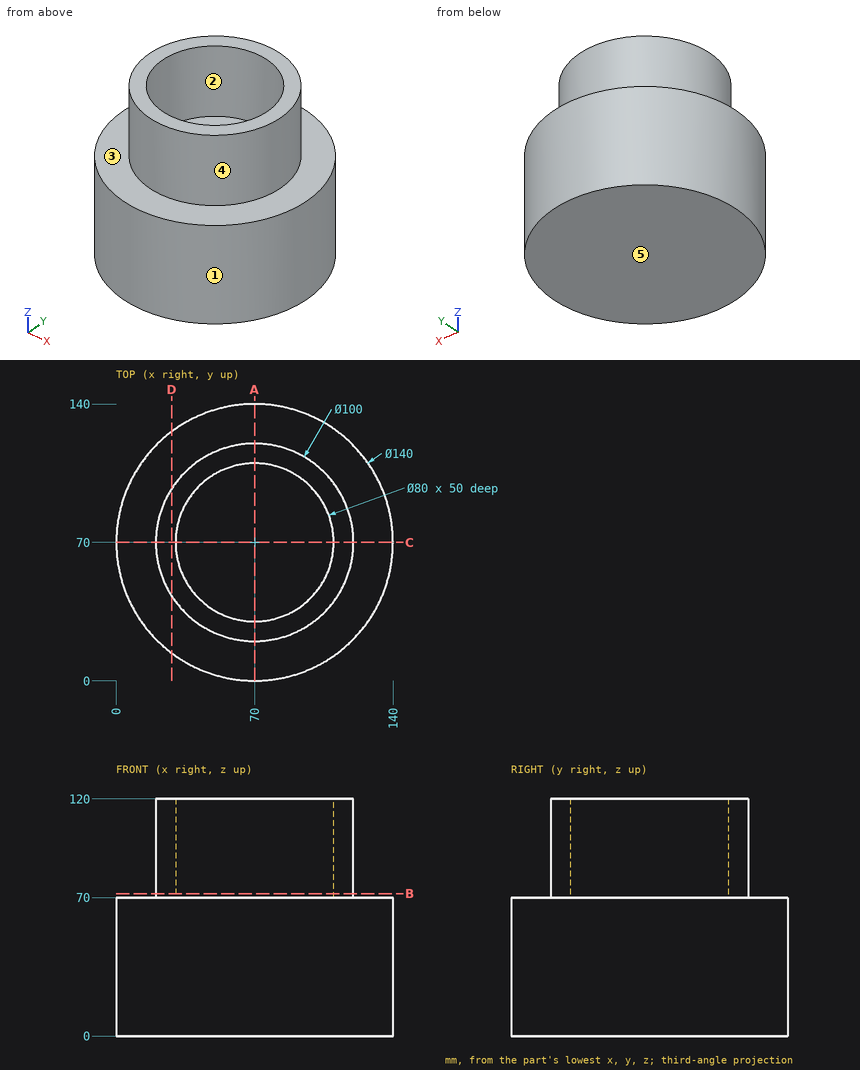
Can you work these out from the drawing? Everything is in mm from the part's minimum corner. A direction names the side the tool comes from. Round coordinates to 2 decimals unless told otherwise and drop trailing zeros. Write each loop counter-clockwise with the first axis right and the second up, starting at its lowest first coordinate (ties: lowest second). Pieces come first, ordered by that corner, then holes.
1. Will these pins go through, and if not, where does the flat tip stop? pin 1 Ø4 at (x, z) = (111.5, 60.5) entering from -Y; pin 2 Ø10 at (x, y) = (48, 78) entering from +Z; pin 3 Ø8 at (x, z) = (26.5, 92.5) entering from +Y.
2. Suppose I cut it at B-B (z = 72). List the corners of the cut face in (x, y) for me, and give its area (3 significant figures).
3. I need wall thicknesses on L1, parallel to Y at x = 70, z = 93; L2, parallel to Z at x = 71, y = 132; L3, parallel to X at y = 49, z = 87.5. Which ranges of each line are inside material? Lowest first, please.
4. If we mould it in two halves opening along Y, with no side actions, what happens to the marked faces 1, 2 and 3? For each: released by +Y, released by -Y, zero draft, split by the parting line, or undercut.
5. Suppose I cut it at D-D (x = 28). List the corners of the cut face in (y, z) for me, and give its area (3 significant figures).
6. For the marked faces 4 and 5, which set-ups out of +Z, -Z, +X, -X, +Y, -Y let a thin tool reach every point of the face, with its end or its side?
7. Suppose I cut it at A-A (x = 70). List the corners of the cut face in (y, z) for me.
Answer sheet:
1. pin 1: stops at y = 12.21
1. pin 2: stops at z = 70
1. pin 3: stops at y = 100.66
2. outline: circle Ø100 at (70, 70); hole circle Ø80 at (70, 70)
2. area: 2,830 mm2
3. L1: y = 20 to 30, 110 to 120
3. L2: z = 0 to 70
3. L3: x = 24.62 to 35.96, 104.04 to 115.38
4. face 1: split by the parting line
4. face 2: undercut
4. face 3: zero draft
5. outline: (14, 0) - (126, 0) - (126, 70) - (97.13, 70) - (97.13, 120) - (42.87, 120) - (42.87, 70) - (14, 70) - close
5. area: 10,600 mm2
6. face 4: +Z
6. face 5: -Z, +X, -X, +Y, -Y
7. outline: (0, 0) - (140, 0) - (140, 70) - (120, 70) - (120, 120) - (110, 120) - (110, 70) - (30, 70) - (30, 120) - (20, 120) - (20, 70) - (0, 70) - close
